```python
from build123d import *

# Parameters (mm, degrees)
F0_W     = 38.1
F0_H     = 44.45
F1_DEPTH = 12.7
F2_R     = 5.08
F3_R     = 2.54
F4_DEPTH = 38.1
F5_R     = 2.54
F6_DEPTH = 6.35


with BuildPart() as f1:
    # F0 (on Front) → F1 (new body)
    with BuildSketch(Plane.XZ):
        with Locations((-19.05, 5.328478)):
            Rectangle(F0_W, F0_H)
    extrude(amount=F1_DEPTH)

    # F2
    f2_edges = [f1.edges().sort_by_distance(p)[0] for p in [
        (-19.05, 0, -16.896522),
        (-19.05, -12.7, -16.896522),
    ]]
    fillet(f2_edges, radius=F2_R)

    # F3 (on face) → F4 (cut)
    with BuildSketch(Plane.YZ):
        with Locations((-6.35, -10.546522)):
            Circle(F3_R)
        with Locations((-6.35, 21.203478)):
            Circle(F3_R)
    extrude(amount=-F4_DEPTH, mode=Mode.SUBTRACT)

    # F5 (on face) → F6 (cut)
    with BuildSketch(Plane.XY.offset(27.553478)):
        with Locations((-19.05, -6.35)):
            Circle(F5_R)
    extrude(amount=-F6_DEPTH, mode=Mode.SUBTRACT)


solid = f1.part
```
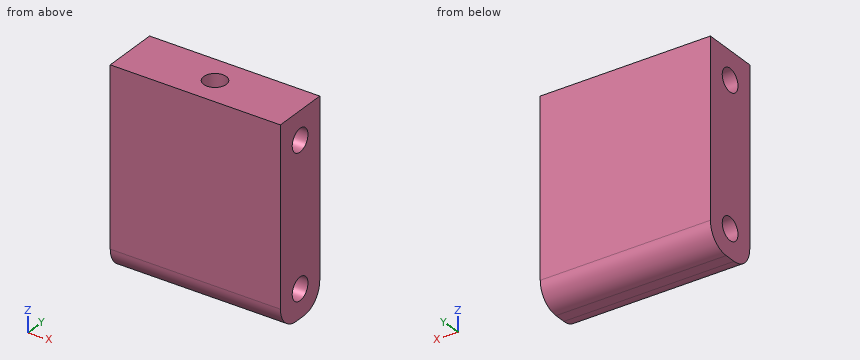
Work out the finished part from the listing and answer in its coordinate system (mm). Round coordinates to 2 decimals unless told otherwise and drop trailing zeros. Order: outer loops, then holes, each group sorted by start corner. A loop starts at its lowest first (then second) coordinate and runs counter-clockwise, first axis right, second up.
Q1. A cutting plane is placed at B-B, the plane z = 20.5. Determine the outline of the cut face in (x, y), then the cut area to 3 significant figures.
Solution:
outline: (-38.1, -12.7) - (0, -12.7) - (0, -8.79) - (-38.1, -8.79) - close; (-38.1, -3.91) - (0, -3.91) - (0, 0) - (-38.1, 0) - close
area: 298 mm2
Q2. Find the intervals of material crossed by line 1 along Z through (x, y) = (-27, -6.35); line 2 along Z through (x, y) = (-24, -7.5); line 3 along Y through (x, z) = (-19, 26), in increasing order.
Solution:
line 1: z = -16.9 to -13.09, -8.01 to 18.66, 23.74 to 27.55
line 2: z = -16.9 to -12.81, -8.28 to 18.94, 23.47 to 27.55
line 3: y = -12.7 to -8.89, -3.81 to 0
Q3. A cutting plane is placed at C-C, the plane x = -19.05. Determine the outline of the cut face in (y, z).
Solution:
outline: (-12.7, -11.82) arc R5.08 ccw to (-7.62, -16.9) - (-5.08, -16.9) arc R5.08 ccw to (0, -11.82) - (0, 27.55) - (-3.81, 27.55) - (-3.81, 21.2) arc R2.54 cw to (-8.89, 21.2) - (-8.89, 27.55) - (-12.7, 27.55) - close; hole circle Ø5.08 at (-6.35, -10.55)
Q4. A cutting plane is placed at D-D, the plane x = -8. Determine the outline of the cut face in (y, z).
Solution:
outline: (-12.7, -11.82) arc R5.08 ccw to (-7.62, -16.9) - (-5.08, -16.9) arc R5.08 ccw to (0, -11.82) - (0, 27.55) - (-12.7, 27.55) - close; hole circle Ø5.08 at (-6.35, -10.55); hole circle Ø5.08 at (-6.35, 21.2)
Q5. A cutting plane is placed at A-A, the plane y = -6.35. Determine the outline of the cut face in (x, z), then the cut area to 3 significant figures.
Solution:
outline: (-38.1, -16.9) - (0, -16.9) - (0, -13.09) - (-38.1, -13.09) - close; (-38.1, -8.01) - (0, -8.01) - (0, 18.66) - (-38.1, 18.66) - close; (-38.1, 23.74) - (-21.59, 23.74) - (-21.59, 27.55) - (-38.1, 27.55) - close; (-16.51, 23.74) - (0, 23.74) - (0, 27.55) - (-16.51, 27.55) - close
area: 1,290 mm2
